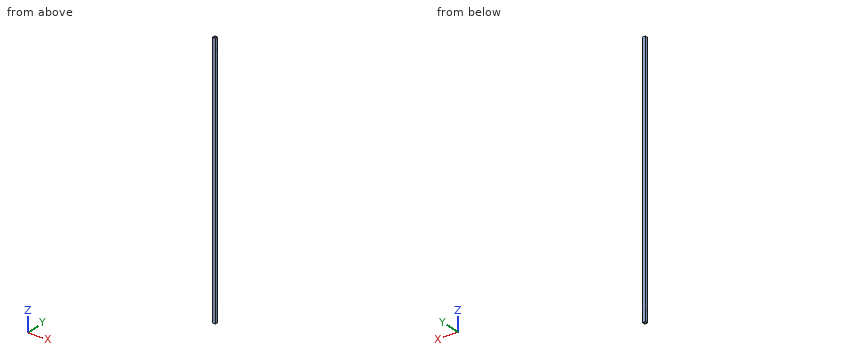
from build123d import *

# Parameters (mm, degrees)
SKETCH_1_W          = 20
SKETCH_1_H          = 20
SKETCH_1_W_2        = 18
SKETCH_1_H_2        = 18
EXTRUDE_1_DEPTH     = 1820
SKETCH_2_R          = 2
CUT_EXTRUDE_1_DEPTH = 1821.219766951


with BuildPart() as part:
    # 草图1 → 凸台-拉伸1 (new body)
    with BuildSketch(Plane.XY):
        with Locations((10, 10)):
            Rectangle(SKETCH_1_W, SKETCH_1_H)
        with Locations((10, 10)):
            Rectangle(SKETCH_1_W_2, SKETCH_1_H_2, mode=Mode.SUBTRACT)
    extrude(amount=EXTRUDE_1_DEPTH)

    # 草图2 → 切除-拉伸1 (cut, through all)
    with BuildSketch(Plane.ZY):
        with Locations((1812.8, 5)):
            Circle(SKETCH_2_R)
        with Locations((1812.8, 15)):
            Circle(SKETCH_2_R)
        with Locations((1752.2, 15)):
            Circle(SKETCH_2_R)
        with Locations((1740.2, 15)):
            Circle(SKETCH_2_R)
        with Locations((1740.2, 5)):
            Circle(SKETCH_2_R)
        with Locations((1752.2, 5)):
            Circle(SKETCH_2_R)
        with Locations((7.2, 5)):
            Circle(SKETCH_2_R)
        with Locations((7.2, 15)):
            Circle(SKETCH_2_R)
        with Locations((67.8, 15)):
            Circle(SKETCH_2_R)
        with Locations((79.8, 15)):
            Circle(SKETCH_2_R)
        with Locations((79.8, 5)):
            Circle(SKETCH_2_R)
        with Locations((67.8, 5)):
            Circle(SKETCH_2_R)
    extrude(amount=-CUT_EXTRUDE_1_DEPTH, mode=Mode.SUBTRACT)


solid = part.part
For this review, take the finished solid that the model builds, in its own axes (mm). Round coordinates to 2 decimals unless told otherwise and drop trailing zeros. Write each loop counter-clockwise with the first axis right and the second up, starting at its lowest first coordinate (ties: lowest second). Pieces come first, ordered by that corner, then holes. Notation, with made-up numbers: (58.5, 67.25) -> (66.5, 67.25) arc R19 ccw to (66.5, 72.25) -> close; hole circle Ø2 at (39, 45.25). An arc over 180 degrees is marked (long way). Use CSV: the item, a comma, the result in double quotes.
(1) Clearance check with a flat-ended pin moving along its axis: P1, Ø5, axis at y = 5, z = 1752.2, coming from the +X side. State where the tip first meets the part, or that it passes through.
Computed values:
P1,"x = 20"
(2) Consider section B-B, the plane z = 731. Give the boundary of the cut face in (x, y).
Computed values:
outline,"(0, 0) -> (20, 0) -> (20, 20) -> (0, 20) -> close; hole (1, 1) -> (19, 1) -> (19, 19) -> (1, 19) -> close"
(3) To check wall thickness, follow L1, parallel to Y at x = 0.35, z = 1752.2; L2, parallel to Y at x = 12.5, z = 367.5. State the ranges of each line that lie inside material, in increasing order. Write a range as [from, to].
Computed values:
L1,"[0, 3], [7, 13], [17, 20]"
L2,"[0, 1], [19, 20]"
(4) Consider section A-A, the plane x = 10.5. Give the boundary of the cut face in (y, z).
Computed values:
outline,"(0, 0) -> (1, 0) -> (1, 1820) -> (0, 1820) -> close; (19, 0) -> (20, 0) -> (20, 1820) -> (19, 1820) -> close"
